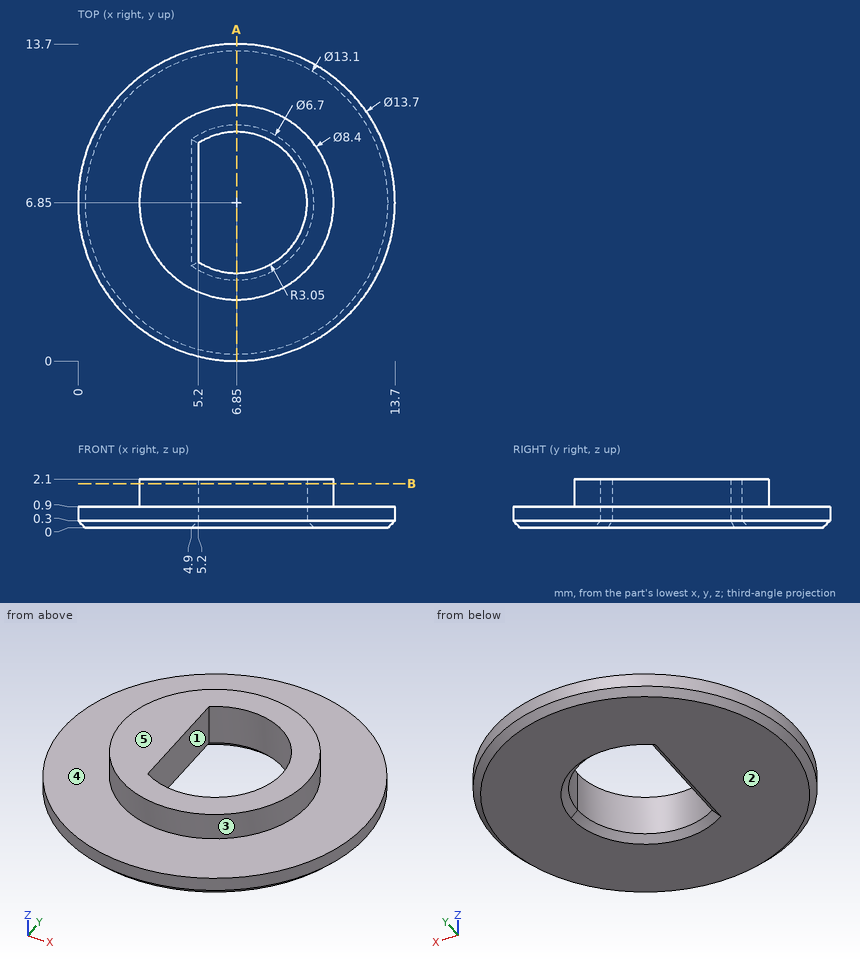
Print and shaded views of the part. All mm, measured from the part's lowest x, y and z. A direction names the side the tool comes from. Coordinates: 2 decimals unless noted, no trailing zeros. Order: outer loops, then holes, each group sorted by start corner. A loop starts at its lowest first (then second) coordinate and runs counter-clockwise, first axis right, second up.
Item 1: Drill centre lines: L1, parallel to Z at x = 1.75, y = 6.25; L2, parallel to Y at x = 7, z = 1.45; L3, parallel to Y at x = 8.75, z = 0.65. Where is each one in solid material? Low to high.
Filled in:
L1: z = 0 to 0.9
L2: y = 2.65 to 3.8, 9.9 to 11.05
L3: y = 0.27 to 4.46, 9.24 to 13.43
Item 2: Tool access for the marked faces 4 and 5: list every direction of +Z, -Z, +X, -X, +Y, -Y with a clear straight run to the whole face (end or side of a thin tool).
Filled in:
face 4: +Z
face 5: +Z, +X, -X, +Y, -Y
Item 3: Mould opens along Y. For the marked faces 1, 2 and 3 say: released by +Y, released by -Y, zero draft, split by the parting line, or undercut.
Filled in:
face 1: undercut
face 2: zero draft
face 3: split by the parting line
Item 4: Saw through at A-A on x = 6.85. List the corners of the cut face in (y, z).
Filled in:
outline: (0, 0.3) - (0.3, 0) - (3.5, 0) - (3.8, 0.3) - (3.8, 2.1) - (2.65, 2.1) - (2.65, 0.9) - (0, 0.9) - close; (9.9, 0.3) - (10.2, 0) - (13.4, 0) - (13.7, 0.3) - (13.7, 0.9) - (11.05, 0.9) - (11.05, 2.1) - (9.9, 2.1) - close
Item 5: Drop a flat-ended pin along its axis: pin 1 Ø0.9 at (y, z) = (5.5, 1.5) entering from +X. Give the stop position or say it passes through.
Filled in:
pin 1: stops at x = 10.95
Item 6: Saw through at B-B on z = 1.9. List the corners of the cut face in (x, y).
Filled in:
outline: circle Ø8.4 at (6.85, 6.85); hole (5.2, 4.28) arc R3.05 ccw (long way) to (5.2, 9.42) - close
